Can you work these out from the model? Positions are in its coordinate system, mm. A direction names the side the tool comes from. Coordinates: 2 decimals unless noted, no trailing zeros. Order: outer loops, then holes, each group sorted by start corner. A loop starts at its lowest first (then second) coordinate and runs counter-clockwise, first axis right, second up. Notation, with made-up numbers: M -33.5,59 L 10.5,59 A21 ccw 10.5,88 Z; hole C 4.5,29.5 d8. An arc over 180 degrees is marked long. Answer as a JSON object with one key per item and string values.
from build123d import *

# Parameters (mm, degrees)
CROQUIS1_W              = 45.4
CROQUIS1_H              = 20.4
SALIENTE_EXTRUIR1_DEPTH = 1.6
CROQUIS2_R              = 0.7
CORTAR_EXTRUIR1_DEPTH   = 1
SALIENTE_EXTRUIR2_DEPTH = 0.5
SALIENTE_EXTRUIR3_DEPTH = 3
CROQUIS9_R              = 7.95
SALIENTE_EXTRUIR4_DEPTH = 11
CROQUIS10_W             = 10
CROQUIS10_H             = 1
SALIENTE_EXTRUIR5_DEPTH = 2
REDONDEO5_R             = 1
CROQUIS13_W             = 9
CROQUIS13_H             = 3
SALIENTE_EXTRUIR6_DEPTH = 1.5
MATRIZL2_COUNT          = 2
MATRIZL2_PITCH          = 18
CROQUIS14_W             = 3
CROQUIS14_H             = 9
SALIENTE_EXTRUIR7_DEPTH = 1.5


with BuildPart() as part:
    # Croquis1 → Saliente-Extruir1 (new body)
    with BuildSketch(Plane(origin=(0, 0, 0), x_dir=(1, 0, 0), z_dir=(0, 1, 0))):
        Rectangle(CROQUIS1_W, CROQUIS1_H)
    extrude(amount=SALIENTE_EXTRUIR1_DEPTH)

    # Croquis2 → Cortar-Extruir1 (cut)
    with BuildSketch(Plane(origin=(0, 1.6, 0), x_dir=(1, 0, 0), z_dir=(0, 1, 0))):
        with Locations(Location((-21.5, 9, 0), (0, 0, 270))):
            Circle(CROQUIS2_R)
        with Locations(Location((21.5, 9, 0), (0, 0, 270))):
            Circle(CROQUIS2_R)
        with Locations(Location((21.5, -9, 0), (0, 0, 270))):
            Circle(CROQUIS2_R)
        with Locations(Location((-21.5, -9, 0), (0, 0, 270))):
            Circle(CROQUIS2_R)
    extrude(amount=-CORTAR_EXTRUIR1_DEPTH, mode=Mode.SUBTRACT)

    # Croquis3 → Saliente-Extruir2 (add)
    with BuildSketch(Plane(origin=(0, 1.6, 0), x_dir=(1, 0, 0), z_dir=(0, 1, 0))):
        with BuildLine():
            Line((-4.202221616, 9.535810589), (4.202221616, 9.535810589))
            ThreePointArc((4.202221616, 9.535810589), (5.818460699, 7.919571506), (4.202221616, 6.303332424))
            Line((4.202221616, 6.303332424), (-4.202221616, 6.303332424))
            ThreePointArc((-4.202221616, 6.303332424), (-5.818460699, 7.919571506), (-4.202221616, 9.535810589))
        make_face()
        with BuildLine():
            Line((-4.202221616, 9.304919292), (4.202221616, 9.304919292))
            ThreePointArc((4.202221616, 9.304919292), (5.587569401, 7.919571506), (4.202221616, 6.534223721))
            Line((4.202221616, 6.534223721), (-4.202221616, 6.534223721))
            ThreePointArc((-4.202221616, 6.534223721), (-5.587569401, 7.919571506), (-4.202221616, 9.304919292))
        make_face(mode=Mode.SUBTRACT)
    extrude(amount=SALIENTE_EXTRUIR2_DEPTH)

    # Croquis8 → Saliente-Extruir3 (add)
    with BuildSketch(Plane(origin=(0, 1.6, 0), x_dir=(1, 0, 0), z_dir=(0, 1, 0))):
        with BuildLine():
            Line((-4.202221616, 9.304919292), (4.202221616, 9.304919292))
            ThreePointArc((4.202221616, 9.304919292), (5.587569401, 7.919571506), (4.202221616, 6.534223721))
            Line((4.202221616, 6.534223721), (-4.202221616, 6.534223721))
            ThreePointArc((-4.202221616, 6.534223721), (-5.587569401, 7.919571506), (-4.202221616, 9.304919292))
        make_face()
    extrude(amount=SALIENTE_EXTRUIR3_DEPTH)

    # Croquis9 → Saliente-Extruir4 (add)
    with BuildSketch(Plane(origin=(0, 1.6, 0), x_dir=(1, 0, 0), z_dir=(0, 1, 0))):
        with Locations(Location((-13.1, 0, 0), (0, 0, 270))):
            Circle(CROQUIS9_R)
        with Locations(Location((13.1, 0, 0), (0, 0, 270))):
            Circle(CROQUIS9_R)
    extrude(amount=SALIENTE_EXTRUIR4_DEPTH)

    # Croquis10 → Saliente-Extruir5 (add)
    with BuildSketch(Plane.XZ):
        with Locations((-0.012747973, 9.7)):
            Rectangle(CROQUIS10_W, CROQUIS10_H)
    extrude(amount=SALIENTE_EXTRUIR5_DEPTH)

    # Redondeo5
    redondeo5_edges = [part.edges().sort_by_distance(p)[0] for p in [
        (-13.1, 12.6, -7.95),
        (13.1, 12.6, -7.95),
    ]]
    fillet(redondeo5_edges, radius=REDONDEO5_R)

    # Croquis13 → Saliente-Extruir6 (add)
    with BuildSketch(Plane.XZ):
        Rectangle(CROQUIS13_W, CROQUIS13_H)
    saliente_extruir6 = extrude(amount=SALIENTE_EXTRUIR6_DEPTH)

    # MatrizL2: Saliente-Extruir6 ×2
    with Locations(*[(i * MATRIZL2_PITCH, 0, 0) for i in range(1, MATRIZL2_COUNT)]):
        add(saliente_extruir6)

    # Croquis14 → Saliente-Extruir7 (add)
    with BuildSketch(Plane.XZ):
        with Locations((-19.2, -0.292211089)):
            Rectangle(CROQUIS14_W, CROQUIS14_H)
    extrude(amount=SALIENTE_EXTRUIR7_DEPTH)


solid = part.part
Item 1: I want a section at A-A, the plane y = -0.5. Write out the boundary of the cut face in (x, z).
Answers follow:
{"outline": "M -20.7,-4.79 L -17.7,-4.79 L -17.7,4.21 L -20.7,4.21 Z; M -5.01,9.2 L 4.99,9.2 L 4.99,10.2 L -5.01,10.2 Z; M -4.5,-1.5 L 4.5,-1.5 L 4.5,1.5 L -4.5,1.5 Z; M 13.5,-1.5 L 22.5,-1.5 L 22.5,1.5 L 13.5,1.5 Z"}
Item 2: Which directions (+Z, -Z, +X, -X, +Y, -Y) give clear straight access to the entire face, cutting with the end or side of a thin tool? Please do faces 1 (the flat face through (22.5, -1, 0)), 2 (the cylindrical face through (-5.818, 1.846, -7.884)), 3 (the flat face through (4.5, -1, 0)), 4 (the flat face through (-19, -1, 4.208)).
Answers follow:
{"face 1": "+Z, -Z, +X, -Y", "face 2": "+Y", "face 3": "-Z, -Y", "face 4": "+Z, +X, -X, -Y"}
Item 3: I want a section at C-C, the plane x = -13.1. Write out the boundary of the cut face in (y, z).
Answers follow:
{"outline": "M 0,-10.2 L 1.6,-10.2 L 1.6,-7.95 L 11.6,-7.95 A1 ccw 12.6,-6.95 L 12.6,6.95 A1 ccw 11.6,7.95 L 1.6,7.95 L 1.6,10.2 L 0,10.2 Z"}
Item 4: If we mould it in two halves opening along X, with no side actions, what happens to faces 5 (the cylindrical face through (-5.587, 3.332, -7.889)), 6 (the flat face through (13, 12.6, 0)), 7 (the cylindrical face through (22.194, 1.107, -9.091)), 8 (the flat face through (-20.7, -1, 0))? For each: pulls with the +X half, pulls with the -X half, needs draft (parallel to the pull), parting line crosses it, or undercut.
Answers follow:
{"face 5": "undercut", "face 6": "needs draft", "face 7": "undercut", "face 8": "pulls with the -X half"}
Item 5: I'm going to push flat-ended pins straight in: pin 1 (1 mm diameter, centred on y = 4, z = -2.5, fed in from +X); pin 2 (2.5 mm diameter, centred on x = 0, y = 3, fed in from +Z); pin 3 (0.5 mm diameter, centred on y = -1.5, z = 9.5, fed in from +X). Where does each tip first touch, or does it pass through?
Answers follow:
{"pin 1": "stops at x = 20.79", "pin 2": "stops at z = -6.3", "pin 3": "stops at x = 4.99"}
Item 6: Please list where these lines run through material, in increasing order: line 1 (X direction, y = 0.95, z = -9); line 2 (X direction, y = -0.5, z = -1); line 3 (Z direction, x = -3, y = -0.75).
Answers follow:
{"line 1": "x = -22.7 to -22.2, -20.8 to 20.8, 22.2 to 22.7", "line 2": "x = -20.7 to -17.7, -4.5 to 4.5, 13.5 to 22.5", "line 3": "z = -1.5 to 1.5, 9.2 to 10.2"}
Item 7: I want a section at B-B, the plane y = 3.5. Write out the boundary of the cut face in (x, z).
Answers follow:
{"outline": "C -13.1,0 d15.9; M -4.2,-9.3 L 4.2,-9.3 A1.39 ccw 4.2,-6.53 L -4.2,-6.53 A1.39 ccw Z; C 13.1,0 d15.9"}
Item 8: I want a section at D-D, the plane z = 0. Write out the boundary of the cut face in (x, y), plus the area to 3 significant figures.
Answers follow:
{"outline": "M -22.7,0 L -20.7,0 L -20.7,-1.5 L -17.7,-1.5 L -17.7,0 L -4.5,0 L -4.5,-1.5 L 4.5,-1.5 L 4.5,0 L 13.5,0 L 13.5,-1.5 L 22.5,-1.5 L 22.5,0 L 22.7,0 L 22.7,1.6 L 21.05,1.6 L 21.05,11.6 A1 ccw 20.05,12.6 L 6.15,12.6 A1 ccw 5.15,11.6 L 5.15,1.6 L -5.15,1.6 L -5.15,11.6 A1 ccw -6.15,12.6 L -20.05,12.6 A1 ccw -21.05,11.6 L -21.05,1.6 L -22.7,1.6 Z", "area": "453 mm^2"}
